The listing builds one solid part. Answer for the finished solid, in the listing's coordinates (mm). Round coordinates to 2 decimals unless told otherwise and drop trailing zeros. Loops run counter-clockwise (first coordinate to the right, second up) from the corner with the lowest first, then second, coordinate; pieces in that order, holes last. Notation, with made-up numbers: (35.5, -22.5) - (76.5, -22.5) arc R25 ccw to (76.5, -7.5) - close; hole circle Ø10 at (35.25, -8). An arc over 180 degrees is marked (long way). One line per item, written item: value.
```python
from build123d import *

# Parameters (mm, degrees)
PAD001_DEPTH = 5
FILLET_R     = 0.3
FILLET001_R  = 0.3


with BuildPart() as part:
    # Sketch002 → Pad001 (new body)
    with BuildSketch(Plane.YZ.offset(29.3)):
        Polygon((5.9, 3.5), (12.8, 3.5), (12.8, 2.4), (12.05, 1.65), (6.65, 1.65), (5.9, 2.4), align=None)
    extrude(amount=PAD001_DEPTH)

    # Fillet
    fillet_edges = [part.edges().sort_by_distance(p)[0] for p in [
        (31.8, 5.9, 3.5),
    ]]
    fillet(fillet_edges, radius=FILLET_R)

    # Fillet001
    fillet001_edges = [part.edges().sort_by_distance(p)[0] for p in [
        (31.8, 12.8, 3.5),
    ]]
    fillet(fillet001_edges, radius=FILLET001_R)


solid = part.part
```
1) A cutting plane is placed at B-B on z = 1.8. Give the vertices of the cut face in (x, y).
Final values:
outline: (29.3, 6.5) - (34.3, 6.5) - (34.3, 12.2) - (29.3, 12.2) - close
2) A cutting plane is placed at C-C on y = 12.25. Give the vertices of the cut face in (x, z), and give its area (3 significant figures).
Final values:
outline: (29.3, 1.85) - (34.3, 1.85) - (34.3, 3.5) - (29.3, 3.5) - close
area: 8.25 mm2
3) Consider L1, parallel to Y at x = 34, z = 2.1; L2, parallel to Y at x = 32.7, z = 1.95. Determine where each line is inside the solid, lowest interval first.
Final values:
L1: 6.2 to 12.5
L2: 6.35 to 12.35
4) A cutting plane is placed at A-A on x = 32.85. Give the vertices of the cut face in (y, z).
Final values:
outline: (5.9, 2.4) - (6.65, 1.65) - (12.05, 1.65) - (12.8, 2.4) - (12.8, 3.2) arc R0.3 ccw to (12.5, 3.5) - (6.2, 3.5) arc R0.3 ccw to (5.9, 3.2) - close
